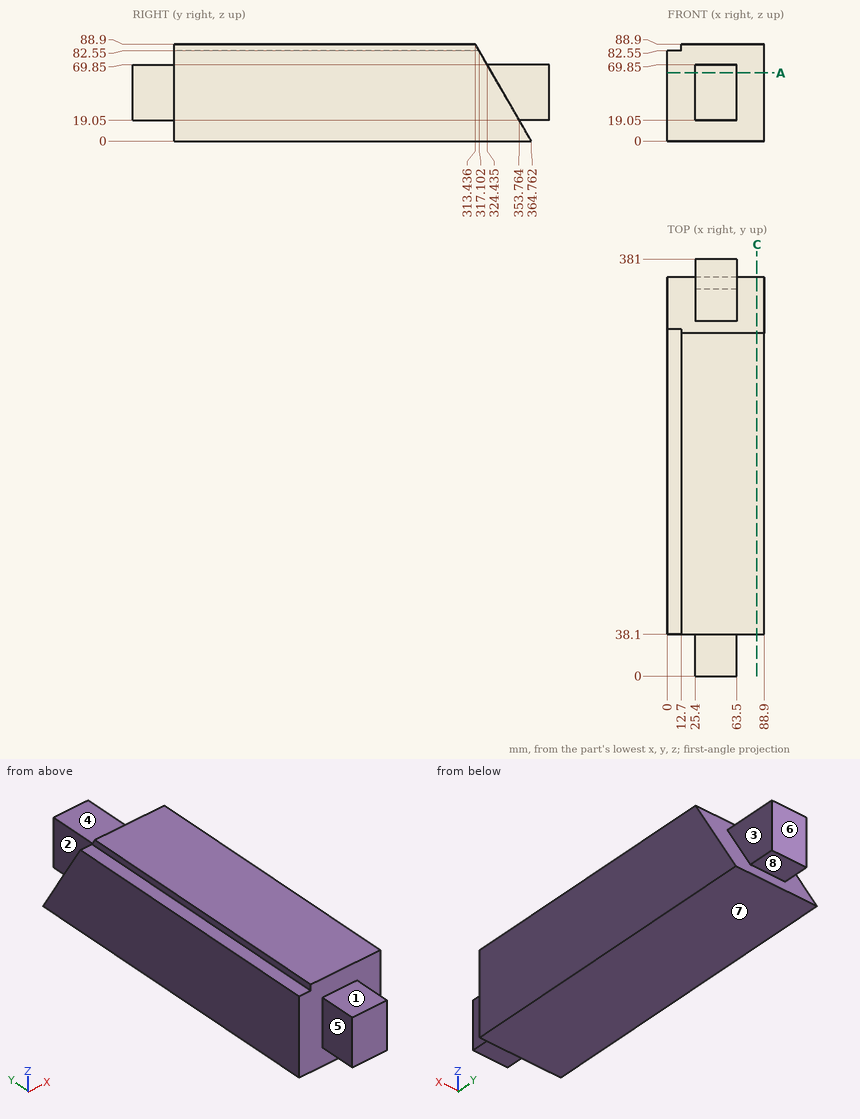
Answer from the drawing. Dimensions are ordinates in mm from the lowest x, y and z of the part. A direction names the side the tool comes from. Give positions to 0.01 mm unless a question says otherwise; leave off trailing zeros. Loops run counter-clockwise (first coordinate to the right, second up) from the corner with the lowest first, then second, coordinate; pieces in that order, holes last. Notation, with made-up numbers: (62.5, 29) - (84.5, 29) arc R30 cw to (84.5, 53) - close; hole circle Ø10 at (-14.75, -38). An arc over 180 degrees is marked (long way). Answer as a JSON object with one key per item and string values.
1. Flat-ended cylindrical pins translate along their axes: pin 1 Ø11.5 at (x, y) = (48, 365) entering from +Z; pin 2 Ø19 at (x, y) = (46, 19) entering from -Z; pin 3 Ø3 at (x, z) = (14.5, 56.5) entering from -Y. Find the tip coordinate at first contact, or state that the pin passes through.
Determined:
{"pin 1": "z = 69.85", "pin 2": "z = 19.05", "pin 3": "y = 38.1"}
2. For the marked faces 1, 2, 3, 4 and 5, determine the directions among +Z, -Z, +X, -X, +Y, -Y from which every point of the face is accessible in a straight line to the end or side of a thin tool.
Determined:
{"face 1": "+Z, +X, -X, -Y", "face 2": "+Z, -X, +Y", "face 3": "+Z, +X, +Y", "face 4": "+Z, +X, -X, +Y", "face 5": "+Z, -Z, -X, -Y"}
3. A cutting plane is placed at C-C (x = 82). Write down the section's boundary in (y, z).
Determined:
{"outline": "(38.1, 0) - (364.76, 0) - (313.44, 88.9) - (38.1, 88.9) - close"}
4. Find the intervals of material crossed by L1, parallel to Z at x = 4.5, y = 230; L2, parallel to X at y = 360, z = 65.5; L3, parallel to Z at x = 24.5, y = 319.5 (1 decimal), in increasing order. Write a range as [from, to].
Determined:
{"L1": "[0, 82.55]", "L2": "[25.4, 63.5]", "L3": "[0, 78.4]"}
5. For a pull along Z with two mould halves and no side action, classify the marked faces 6, 7 and 8 as pulls with the +Z half, pulls with the -Z half, needs draft (parallel to the pull), parting line crosses it, or undercut.
Determined:
{"face 6": "needs draft", "face 7": "pulls with the -Z half", "face 8": "undercut"}
6. A cutting plane is placed at A-A (z = 62.5). Write down the section's boundary in (x, y), then the cut area to 3 significant figures.
Determined:
{"outline": "(0, 38.1) - (25.4, 38.1) - (25.4, 0) - (63.5, 0) - (63.5, 38.1) - (88.9, 38.1) - (88.9, 328.68) - (63.5, 328.68) - (63.5, 381) - (25.4, 381) - (25.4, 328.68) - (0, 328.68) - close", "area": "29,300 mm²"}
